For this review, take the finished solid that the model builds, in its own axes (mm). Face numbers are marked on the shaded views. A direction names the side the tool comes from. Give positions to 0.01 mm unless a question says otherwise; leave off trailing zeros. Loops run counter-clockwise (first coordinate to the right, second up) from the corner with the lowest first, then second, coordinate; pieces in that order, holes last. Notation, with made-up numbers: (87, -33) - (136, -33) arc R30 cw to (136, -11) - close; hole circle Ø11 at (86, 12). An arc over 180 degrees is marked (long way). Answer in a Markdown table with one row per item.
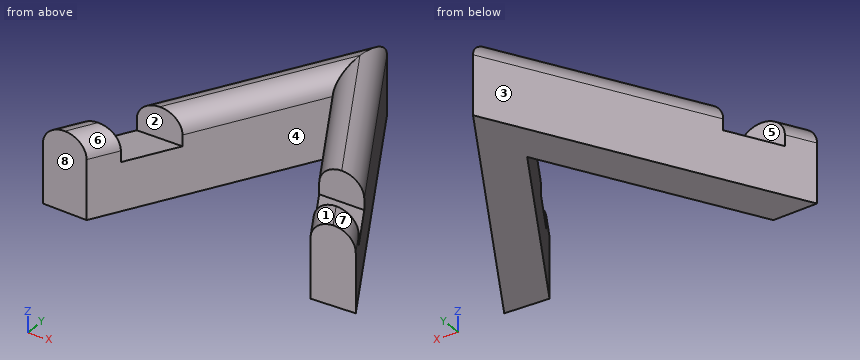
```python
from build123d import *

# Parameters (mm, degrees)
F1_DEPTH = 10
F2_W     = 48.9705931395
F2_H     = 6.2394971028
F3_DEPTH = 3.9
F4_R     = 2.49999


# Not quite as in the source:
# - a fillet or chamfer is up to 0.001 mm smaller than in the source, because OpenCascade refuses the exact size


with BuildPart() as f1:
    # F0 (on Top) → F1 (new body)
    with BuildSketch(Plane.XY):
        Polygon((-14.5670969574, -24.9256566167), (0, 0), (13.7898046523, -24.9256566167), (19.3909112023, -24.7212815966), (0.1191440202, 10.1132547357), (-20.2359139567, -24.7161410615), align=None)
    extrude(amount=F1_DEPTH)

    # F2 (on face) → F3 (cut)
    with BuildSketch(Plane.XY.offset(10)):
        with Locations((2.1743709221, -18.3403375559)):
            Rectangle(F2_W, F2_H)
    extrude(amount=-F3_DEPTH, mode=Mode.SUBTRACT)

    # F4 (radius 2.5 in the source; OpenCascade refuses exactly that, so slightly less here)
    f4_edges = [f1.edges().sort_by_distance(p)[0] for p in [
        (-7.283681, -2.553667, 10),
        (7.126959, -2.553667, 10),
        (-4.447622, -7.610295, 10),
        (4.210299, -7.610295, 10),
        (-19.284459, -23.088114, 10),
        (-13.554419, -23.192871, 10),
        (12.831163, -23.192871, 10),
        (18.488804, -23.090684, 10),
    ]]
    fillet(f4_edges, radius=F4_R)


solid = f1.part
```
1. We need section A-A, the plane y = -16.5. Give the boundary of the cut face in (x, z).
Values:
| item | result |
|---|---|
| outline | (-15.43, 0) - (-9.64, 0) - (-9.64, 6.1) - (-15.43, 6.1) - close; (9.13, 0) - (14.84, 0) - (14.84, 6.1) - (9.13, 6.1) - close |
2. We need section B-B, the plane z = 2.5. Give the boundary of the cut face in (x, y), and give its area (3 significant figures).
Values:
| item | result |
|---|---|
| outline | (-20.24, -24.72) - (-14.57, -24.93) - (0, 0) - (13.79, -24.93) - (19.39, -24.72) - (0.12, 10.11) - close |
| area | 344 mm^2 |
3. For the marked faces 4, 5, 6, 7 and 8, list the 3-axis set-ups (+Z, -Z, +X, -X, +Y, -Y) from which the entire face can be reached by the end or side of a thin tool; tool diameter is ignored.
Values:
| item | result |
|---|---|
| face 4 | +Z, -Z, -Y |
| face 5 | +Z, +X, -X |
| face 6 | +Z, -Y |
| face 7 | +Z, +X, +Y |
| face 8 | +Z, -Z, -X, -Y |
4. Clearance check with flat-ended pins moving along their axes: pin 1 (4.5 mm diameter, centred on x = -12, z = 8, fed in from -Y); pin 2 (3 mm diameter, centred on x = 11.5, z = 9, fed in from +Y); pin 3 (2 mm diameter, centred on y = -18.5, z = 2.5, fed in from -X). State where each tip first meets the part, or that it passes through.
Values:
| item | result |
|---|---|
| pin 1 | stops at y = -24.33 |
| pin 2 | stops at y = -8.32 |
| pin 3 | stops at x = -17.19 |
5. Mouldability with a two-part tool opening along Y and no side actions: class the marked faces 1, 2 and 3 as released by +Y, released by -Y, zero draft, split by the parting line, or undercut.
Values:
| item | result |
|---|---|
| face 1 | released by -Y |
| face 2 | undercut |
| face 3 | released by +Y |
6. Wall thickness on line 1 (Y direction, x = 12.5, z = 7.5); line 2 (X direction, y = -1, z = 1.75); line 3 (X direction, y = -15, z = 2.25): over which ranges is each line inside the solid? List them lowest first. Write a range as [from, to].
Values:
| item | result |
|---|---|
| line 1 | y = [-22.59, -21.46], [-15.22, -12.27] |
| line 2 | x = [-6.38, -0.58], [0.55, 6.27] |
| line 3 | x = [-14.56, -8.77], [8.3, 14.01] |
